Here's how the part is built. I have some questions about the finished solid (model axes, mm). Face numbers are marked on the shaded views. A direction names the side the tool comes from. Coordinates: 2 decimals unless noted, no trailing zeros. Write each loop counter-clockwise with the first axis right and the second up, starting at its lowest first coordinate (ties: lowest second). Pieces come first, ordered by that corner, then holes. Notation, with made-up numbers: (-17.5, -31) - (15.5, -31) arc R16 ccw to (15.5, -14) - close; hole circle Ø3 at (-20.5, 47). An arc over 180 degrees is marked (long way). Answer in a Markdown table with one row per item. Add a question column.
Item 1: Imagine slicing it at C-C (z = 17.5). State how many separate pieces and enclosed holes the cut face has, plus the area to 3 significant figures.
Item 2: Which directions (+Z, -Z, +X, -X, +Y, -Y) give clear straight access to the entire face, cutting with the end or side of a thin tool? Please do the marked faces 1 and 2.
Item 3: Imagine slicing it at A-A (x = -2.5). Please give me the cut outline in (y, z), plus the area to 3 significant figures.
Item 4: I'm going to push flat-ended pins straight in: pin 1 (12 mm diameter, centred on y = 0.5, z = -21.5, fed in from +X); pin 2 (8 mm diameter, centred on x = 20.5, y = 13, fed in from -Z); pin 3 (8 mm diameter, centred on x = 20.5, z = 34.5, fed in from +Y). Where does each tip first touch, or does it pass through?
Item 5: Imagine slicing it at B-B (y = -1). Please give me the cut outline in (x, z).
Item 6: We'd pull the mould along X, two halves only. Please class the marked faces 3 and 4: +X half, -X half, draft (parallel to the pull), parting line (faces both ways), or undercut.
Item 7: If I drill on probe 1 along X at (y, z) = (-2.5, 33); probe 2 along Y at (x, z) = (-36, -6.5); probe 3 along X at (y, z) = (-13.5, 30.5), over which ranges is the centre line in solid material (lowest first)? Write a range as from..to.
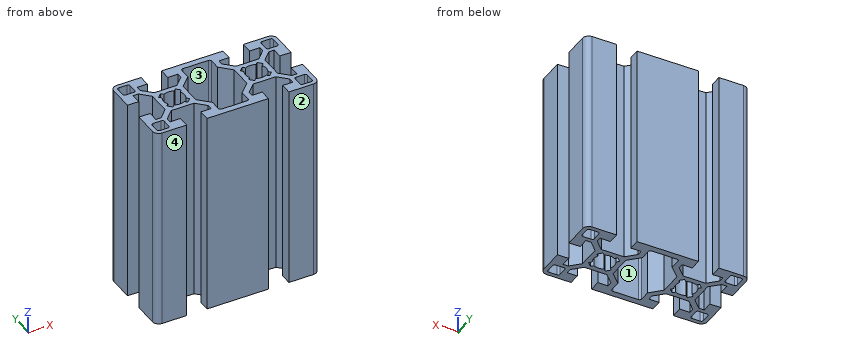
from build123d import *

# Parameters (mm, degrees)
BOSS_EXTRUDE1_DEPTH = 50


with BuildPart() as part:
    # Sketch1 → Boss-Extrude1 (new, symmetric)
    with BuildSketch(Plane.XY):
        with BuildLine():
            Line((-15, -20), (15, -20))
            Line((15, -20), (15, -14.5))
            Line((15, -14.5), (10, -14.5))
            Line((10, -14.5), (10, -11.944543648))
            Line((10, -11.944543648), (14.444543648, -7.5))
            Line((14.444543648, -7.5), (25.555456352, -7.5))
            Line((25.555456352, -7.5), (30, -11.944543648))
            Line((30, -11.944543648), (30, -14.5))
            Line((30, -14.5), (25, -14.5))
            Line((25, -14.5), (25, -20))
            Line((25, -20), (37, -20))
            ThreePointArc((37, -20), (39.121320344, -19.121320344), (40, -17))
            Line((40, -17), (40, -5))
            Line((40, -5), (34.5, -5))
            Line((34.5, -5), (34.5, -10))
            Line((34.5, -10), (31.944543648, -10))
            Line((31.944543648, -10), (27.5, -5.555456352))
            Line((27.5, -5.555456352), (27.5, 5.555456352))
            Line((27.5, 5.555456352), (31.944543648, 10))
            Line((31.944543648, 10), (34.5, 10))
            Line((34.5, 10), (34.5, 5))
            Line((34.5, 5), (40, 5))
            Line((40, 5), (40, 17))
            ThreePointArc((40, 17), (39.121320344, 19.121320344), (37, 20))
            Line((37, 20), (25, 20))
            Line((25, 20), (25, 14.5))
            Line((25, 14.5), (30, 14.5))
            Line((30, 14.5), (30, 11.944543648))
            Line((30, 11.944543648), (25.555456352, 7.5))
            Line((25.555456352, 7.5), (14.444543648, 7.5))
            Line((14.444543648, 7.5), (10, 11.944543648))
            Line((10, 11.944543648), (10, 14.5))
            Line((10, 14.5), (15, 14.5))
            Line((15, 14.5), (15, 20))
            Line((15, 20), (-15, 20))
            Line((-15, 20), (-15, 14.5))
            Line((-15, 14.5), (-10, 14.5))
            Line((-10, 14.5), (-10, 11.944543648))
            Line((-10, 11.944543648), (-14.444543648, 7.5))
            Line((-14.444543648, 7.5), (-25.555456352, 7.5))
            Line((-25.555456352, 7.5), (-30, 11.944543648))
            Line((-30, 11.944543648), (-30, 14.5))
            Line((-30, 14.5), (-25, 14.5))
            Line((-25, 14.5), (-25, 20))
            Line((-25, 20), (-37, 20))
            ThreePointArc((-37, 20), (-39.121320344, 19.121320344), (-40, 17))
            Line((-40, 17), (-40, 5))
            Line((-40, 5), (-34.5, 5))
            Line((-34.5, 5), (-34.5, 10))
            Line((-34.5, 10), (-31.944543648, 10))
            Line((-31.944543648, 10), (-27.5, 5.555456352))
            Line((-27.5, 5.555456352), (-27.5, -5.555456352))
            Line((-27.5, -5.555456352), (-31.944543648, -10))
            Line((-31.944543648, -10), (-34.5, -10))
            Line((-34.5, -10), (-34.5, -5))
            Line((-34.5, -5), (-40, -5))
            Line((-40, -5), (-40, -17))
            ThreePointArc((-40, -17), (-39.121320344, -19.121320344), (-37, -20))
            Line((-37, -20), (-25, -20))
            Line((-25, -20), (-25, -14.5))
            Line((-25, -14.5), (-30, -14.5))
            Line((-30, -14.5), (-30, -11.944543648))
            Line((-30, -11.944543648), (-25.555456352, -7.5))
            Line((-25.555456352, -7.5), (-14.444543648, -7.5))
            Line((-14.444543648, -7.5), (-10, -11.944543648))
            Line((-10, -11.944543648), (-10, -14.5))
            Line((-10, -14.5), (-15, -14.5))
            Line((-15, -14.5), (-15, -20))
        make_face()
        with BuildLine():
            Line((-38, 13), (-38, 17))
            ThreePointArc((-38, 17), (-37.707106781, 17.707106781), (-37, 18))
            Line((-37, 18), (-33, 18))
            ThreePointArc((-33, 18), (-32.292893219, 17.707106781), (-32, 17))
            Line((-32, 17), (-32, 13))
            ThreePointArc((-32, 13), (-32.292893219, 12.292893219), (-33, 12))
            Line((-33, 12), (-37, 12))
            ThreePointArc((-37, 12), (-37.707106781, 12.292893219), (-38, 13))
        make_face(mode=Mode.SUBTRACT)
        with BuildLine():
            Line((-15.555022098, -2.500434253), (-14.423651249, -3.631805103))
            Line((-14.423651249, -3.631805103), (-16.368194897, -5.576348751))
            Line((-16.368194897, -5.576348751), (-17.499565747, -4.444977902))
            ThreePointArc((-17.499565747, -4.444977902), (-20, -5.1), (-22.500434253, -4.444977902))
            Line((-22.500434253, -4.444977902), (-23.631805103, -5.576348751))
            Line((-23.631805103, -5.576348751), (-25.576348751, -3.631805103))
            Line((-25.576348751, -3.631805103), (-24.444977902, -2.500434253))
            ThreePointArc((-24.444977902, -2.500434253), (-25.1, 0), (-24.444977902, 2.500434253))
            Line((-24.444977902, 2.500434253), (-25.576348751, 3.631805103))
            Line((-25.576348751, 3.631805103), (-23.631805103, 5.576348751))
            Line((-23.631805103, 5.576348751), (-22.500434253, 4.444977902))
            ThreePointArc((-22.500434253, 4.444977902), (-20, 5.1), (-17.499565747, 4.444977902))
            Line((-17.499565747, 4.444977902), (-16.368194897, 5.576348751))
            Line((-16.368194897, 5.576348751), (-14.423651249, 3.631805103))
            Line((-14.423651249, 3.631805103), (-15.555022098, 2.500434253))
            ThreePointArc((-15.555022098, 2.500434253), (-14.9, 0), (-15.555022098, -2.500434253))
        make_face(mode=Mode.SUBTRACT)
        with BuildLine():
            Line((-38, -17), (-38, -13))
            ThreePointArc((-38, -13), (-37.707106781, -12.292893219), (-37, -12))
            Line((-37, -12), (-33, -12))
            ThreePointArc((-33, -12), (-32.292893219, -12.292893219), (-32, -13))
            Line((-32, -13), (-32, -17))
            ThreePointArc((-32, -17), (-32.292893219, -17.707106781), (-33, -18))
            Line((-33, -18), (-37, -18))
            ThreePointArc((-37, -18), (-37.707106781, -17.707106781), (-38, -17))
        make_face(mode=Mode.SUBTRACT)
        with BuildLine():
            Line((38, -13), (38, -17))
            ThreePointArc((38, -17), (37.707106781, -17.707106781), (37, -18))
            Line((37, -18), (33, -18))
            ThreePointArc((33, -18), (32.292893219, -17.707106781), (32, -17))
            Line((32, -17), (32, -13))
            ThreePointArc((32, -13), (32.292893219, -12.292893219), (33, -12))
            Line((33, -12), (37, -12))
            ThreePointArc((37, -12), (37.707106781, -12.292893219), (38, -13))
        make_face(mode=Mode.SUBTRACT)
        with BuildLine():
            Line((15.555022098, 2.500434253), (14.423651249, 3.631805103))
            Line((14.423651249, 3.631805103), (16.368194897, 5.576348751))
            Line((16.368194897, 5.576348751), (17.499565747, 4.444977902))
            ThreePointArc((17.499565747, 4.444977902), (20, 5.1), (22.500434253, 4.444977902))
            Line((22.500434253, 4.444977902), (23.631805103, 5.576348751))
            Line((23.631805103, 5.576348751), (25.576348751, 3.631805103))
            Line((25.576348751, 3.631805103), (24.444977902, 2.500434253))
            ThreePointArc((24.444977902, 2.500434253), (25.1, 0), (24.444977902, -2.500434253))
            Line((24.444977902, -2.500434253), (25.576348751, -3.631805103))
            Line((25.576348751, -3.631805103), (23.631805103, -5.576348751))
            Line((23.631805103, -5.576348751), (22.500434253, -4.444977902))
            ThreePointArc((22.500434253, -4.444977902), (20, -5.1), (17.499565747, -4.444977902))
            Line((17.499565747, -4.444977902), (16.368194897, -5.576348751))
            Line((16.368194897, -5.576348751), (14.423651249, -3.631805103))
            Line((14.423651249, -3.631805103), (15.555022098, -2.500434253))
            ThreePointArc((15.555022098, -2.500434253), (14.9, 0), (15.555022098, 2.500434253))
        make_face(mode=Mode.SUBTRACT)
        with BuildLine():
            Line((38, 17), (38, 13))
            ThreePointArc((38, 13), (37.707106781, 12.292893219), (37, 12))
            Line((37, 12), (33, 12))
            ThreePointArc((33, 12), (32.292893219, 12.292893219), (32, 13))
            Line((32, 13), (32, 17))
            ThreePointArc((32, 17), (32.292893219, 17.707106781), (33, 18))
            Line((33, 18), (37, 18))
            ThreePointArc((37, 18), (37.707106781, 17.707106781), (38, 17))
        make_face(mode=Mode.SUBTRACT)
        with BuildLine():
            Line((6.25, -17), (-6.25, -17))
            ThreePointArc((-6.25, -17), (-6.957106781, -16.707106781), (-7.25, -16))
            Line((-7.25, -16), (-7.25, -10.805456352))
            Line((-7.25, -10.805456352), (-12.5, -5.555456352))
            Line((-12.5, -5.555456352), (-12.5, 5.555456352))
            Line((-12.5, 5.555456352), (-7.25, 10.805456352))
            Line((-7.25, 10.805456352), (-7.25, 16))
            ThreePointArc((-7.25, 16), (-6.957106781, 16.707106781), (-6.25, 17))
            Line((-6.25, 17), (6.25, 17))
            ThreePointArc((6.25, 17), (6.957106781, 16.707106781), (7.25, 16))
            Line((7.25, 16), (7.25, 10.805456352))
            Line((7.25, 10.805456352), (12.5, 5.555456352))
            Line((12.5, 5.555456352), (12.5, -5.555456352))
            Line((12.5, -5.555456352), (7.25, -10.805456352))
            Line((7.25, -10.805456352), (7.25, -16))
            ThreePointArc((7.25, -16), (6.957106781, -16.707106781), (6.25, -17))
        make_face(mode=Mode.SUBTRACT)
    extrude(amount=BOSS_EXTRUDE1_DEPTH, both=True)


solid = part.part
Here are the results:
| question | item | result |
|---|---|---|
| 1 | separate pieces | 1 |
| 1 | enclosed holes | 7 |
| 1 | area | 1,140 mm2 |
| 2 | face 1 | +Z, -Z |
| 2 | face 2 | +Z, -Z, +X, -X, -Y |
| 3 | outline | (-20, -50) - (-17, -50) - (-17, 50) - (-20, 50) - close; (17, -50) - (20, -50) - (20, 50) - (17, 50) - close |
| 3 | area | 600 mm2 |
| 4 | pin 1 | stops at x = 40 |
| 4 | pin 2 | passes through |
| 4 | pin 3 | stops at y = 7.5 |
| 5 | outline | (-27.5, -50) - (-25, -50) - (-25, 50) - (-27.5, 50) - close; (-15, -50) - (-12.5, -50) - (-12.5, 50) - (-15, 50) - close; (12.5, -50) - (15, -50) - (15, 50) - (12.5, 50) - close; (25, -50) - (27.5, -50) - (27.5, 50) - (25, 50) - close |
| 6 | face 3 | undercut |
| 6 | face 4 | draft |
| 7 | probe 1 | x = -27.5..-24.45, -15.55..-12.5, 12.5..15.55, 24.45..27.5 |
| 7 | probe 2 | y = -20..-18, -12..-5, 5..12, 18..20 |
| 7 | probe 3 | x = -40..-38, -32..-30, -10..-7.25, 7.25..10, 30..32, 38..40 |
